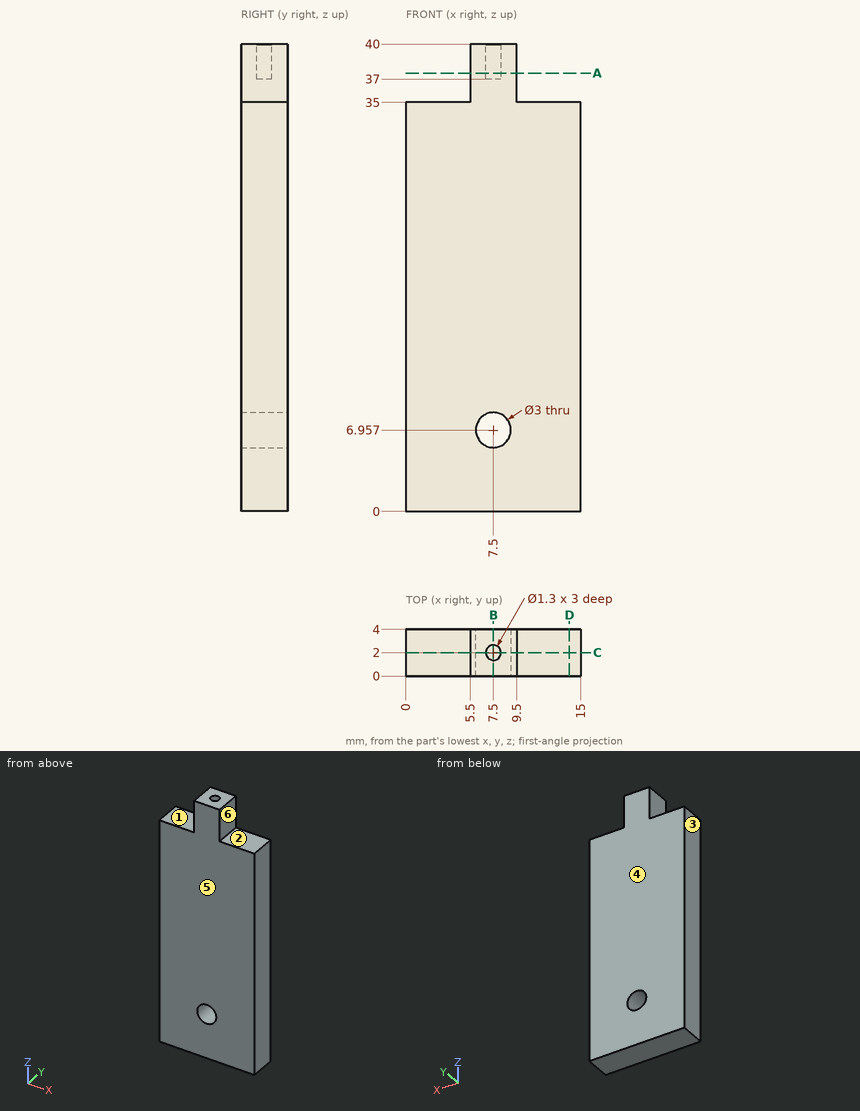
Input: dimensioned drawing with shaded views. Units: mm. Origin: part minimum x, y, z. A direction names the side the tool comes from. Coordinates: 2 decimals unless noted, no trailing zeros. Order: outer loops, then holes, each group sorted by start corner. A loop starts at its lowest first (then second) coordinate and runs counter-clockwise, first axis right, second up. Notation, with made-up numbers: (80, -8.5) - (102, -8.5) arc R4 ccw to (102, -2.5) - close; hole circle Ø11 at (-15, 6.5). An arc over 180 degrees is marked (long way). Return JSON: item names as keys, results as strings. Group by question number.
1. Pull-direction query (Y, two-part tool) for the marked faces 4, 5 and 6; classes: pulls with the +Y half, pulls with the -Y half, needs draft (parallel to the pull), parting line crosses it, or undercut.
2. Cut plane D-D (x = 14). Output: boundary loops of the cut face in (y, z), plus the area to 3 significant figures.
3. Set-up query: the marked faces 1, 2 and 3. Return all of +Z, -Z, +X, -X, +Y, -Y with unobstructed straight access to the full face (end or side cutting, diameter ignored); none if empty.
4. Cut plane A-A (z = 37.5). Output: boundary loops of the cut face in (x, y).
5. Cut plane B-B (x = 7.5). Output: boundary loops of the cut face in (y, z).
6. Pin query (flat end, axial travel): pin 1 (1.2 mm diameter, centred on x = 2.5, y = 2, fed in from +Z); pin 2 (2 mm diameter, centred on y = 3, z = 37.5, fed in from +X). Return the tip coordinate at first contact, or that it passes through.
7. Cut plane C-C (y = 2). Output: boundary loops of the cut face in (x, z), plus the area to 3 significant figures.
8. Material intervals for line 1 along Z through (x, y) = (7.5, 1.5); line 2 along Y through (x, z) = (7.5, 39.2); line 3 along Z through (x, y) = (5.25, 2.75), sorted ascending. Write a range as [from, to].
Resolved:
{
 "1": {"face 4": "pulls with the +Y half", "face 5": "pulls with the -Y half", "face 6": "needs draft"},
 "2": {"outline": "(0, 0) - (4, 0) - (4, 35) - (0, 35) - close", "area": "140 mm²"},
 "3": {"face 1": "+Z, -X, +Y, -Y", "face 2": "+Z, +X, +Y, -Y", "face 3": "+Z, -Z, -X, +Y, -Y"},
 "4": {"outline": "(5.5, 0) - (9.5, 0) - (9.5, 4) - (5.5, 4) - close; hole circle Ø1.3 at (7.5, 2)"},
 "5": {"outline": "(0, 0) - (4, 0) - (4, 5.46) - (0, 5.46) - close; (0, 8.46) - (4, 8.46) - (4, 40) - (2.65, 40) - (2.65, 37) - (1.35, 37) - (1.35, 40) - (0, 40) - close"},
 "6": {"pin 1": "stops at z = 35", "pin 2": "stops at x = 9.5"},
 "7": {"outline": "(0, 0) - (15, 0) - (15, 35) - (9.5, 35) - (9.5, 40) - (8.15, 40) - (8.15, 37) - (6.85, 37) - (6.85, 40) - (5.5, 40) - (5.5, 35) - (0, 35) - close; hole circle Ø3 at (7.5, 6.96)", "area": "534 mm²"},
 "8": {"line 1": "z = [0, 5.46], [8.46, 37]", "line 2": "y = [0, 1.35], [2.65, 4]", "line 3": "z = [0, 35]"}
}
